For this review, take the finished solid that the model builds, in its own axes (mm). Face numbers are marked on the shaded views. A direction names the side the tool comes from. Round coordinates to 2 decimals unless told otherwise and drop trailing zeros. Loops run counter-clockwise (first coordinate to the right, second up) from the corner with the lowest first, then second, coordinate; pieces in that order, holes last.
1. Clearance check with flat-ended pins moving along their axes: pin 1 Ø2 at (x, z) = (1.5, 0) entering from -Y; pin 2 Ø3 at (y, z) = (-24, -1) entering from -X; pin 3 Ø1.5 at (y, z) = (-35.5, -1) entering from +X. State where each tip first meets the part, or that it passes through.
2. To check wall thickness, follow line 1 along Z through (x, y) = (-0.25, -14.5); line 2 along Y through (x, z) = (0.65, -0.65); line 3 along Y through (x, z) = (-0.35, -1.9). State the ranges of each line that lie inside material, in increasing order.
3. Consider section B-B on y = -38. State the section outline as (x, z) points.
4. Consider section A-A on z = 0. State the section outline as (x, y) points.
5. Consider section C-C on x = 0.7. State the section outline as (y, z) points, then the cut area to 3 significant figures.
6. Consider section D-D on y = 19. State the section outline as (x, z) points.
7. Tool access review of the marked faces 1, 2 and 3: name each direction out of +Z, -Z, +X, -X, +Y, -Y from which nothing blocks a thin tool from reaching the whole face with its end or side.
from build123d import *

# Parameters (mm, degrees)
F0_R      = 2.5
F1_DEPTH  = 50
F2_R      = 1.55
F3_DEPTH  = 25
F5_DEPTH  = 42
F7_D      = 3.3
F10_D     = 4.5
F10_DEPTH = 1.4
F10_TIP   = 1.3519363928


with BuildPart() as f1:
    # F0 (on Front) → F1 (new body)
    with BuildSketch(Plane.XZ):
        Circle(F0_R)
    extrude(amount=F1_DEPTH)

    # F2 (on face) → F3 (join)
    with BuildSketch(Plane(origin=(0, 0, 0), x_dir=(-1, 0, 0), z_dir=(0, 1, 0))):
        Circle(F2_R)
    extrude(amount=F3_DEPTH)

    # F4 (on face) → F5 (cut)
    with BuildSketch(Plane.XZ.offset(50)):
        with BuildLine():
            ThreePointArc((2.5, 0), (1.767766953, 1.767766953), (0, 2.5))
            Line((0, 2.5), (0, -2.5))
            ThreePointArc((0, -2.5), (1.767766953, -1.767766953), (2.5, 0))
        make_face()
    extrude(amount=-F5_DEPTH, mode=Mode.SUBTRACT)

    # F7 (through all)
    with Locations(Plane.YZ):
        with Locations((-34.5, 0), (-14.5, 0)):
            Hole(F7_D / 2)

    # F10
    with Locations(Plane(origin=(-2.5, 0, 0), x_dir=(0, 1, 0), z_dir=(-1, 0, 0))):
        with Locations((-34.4858653843, 0), (-14.4858653843, 0)):
            Hole(F10_D / 2, depth=F10_DEPTH)
            with Locations((0, 0, -(F10_DEPTH + F10_TIP / 2))):  # 118° drill point
                Cone(0, F10_D / 2, F10_TIP, mode=Mode.SUBTRACT)


solid = f1.part
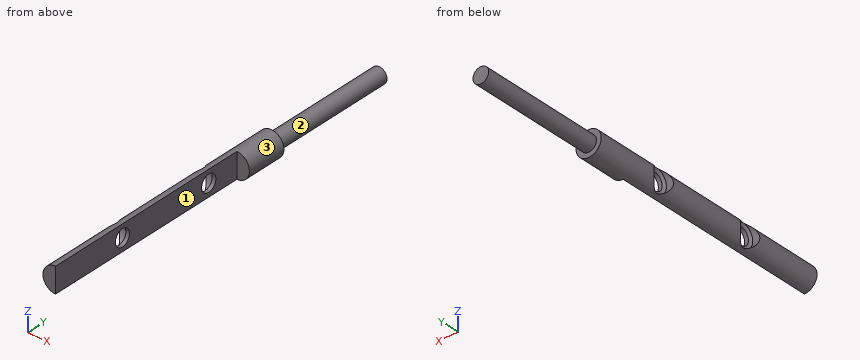
Resolved:
1. pin 1: stops at y = -8
1. pin 2: stops at x = -2.5
1. pin 3: stops at x = 0
2. line 1: z = -2.49 to -1.65, 1.65 to 2.49
2. line 2: y = -8 to 25
2. line 3: y = -50 to 0
3. outline: (0, -2.5) - (0, 2.5) arc R2.5 ccw to start
4. outline: (-2.5, -50) - (0, -50) - (0, -36.15) - (-0.75, -36.15) - (-1.1, -36.74) - (-2.5, -36.74) - close; (-2.5, -32.24) - (-1.1, -32.24) - (-0.73, -32.85) - (0, -32.85) - (0, -16.15) - (-0.75, -16.15) - (-1.1, -16.74) - (-2.5, -16.74) - close; (-2.5, -12.24) - (-1.1, -12.24) - (-0.73, -12.85) - (0, -12.85) - (0, -8) - (2.5, -8) - (2.5, 0) - (1.55, 0) - (1.55, 25) - (-1.55, 25) - (-1.55, 0) - (-2.5, 0) - close
5. outline: (-8, -2.4) - (0, -2.4) - (0, -1.38) - (25, -1.38) - (25, 1.38) - (0, 1.38) - (0, 2.4) - (-8, 2.4) - close
5. area: 108 mm2
6. outline: circle Ø3.1 at (0, 0)
7. face 1: +Z, -Z, +X, -Y
7. face 2: +Y
7. face 3: +Y, -Y
